Build history of the part. All positions in model axes, mm. Face numbers are marked on the shaded views. A direction names the side the tool comes from. Round coordinates to 2 decimals unless told otherwise and drop trailing zeros. Order: outer loops, then holes, each group sorted by start corner. A loop starts at its lowest first (then second) coordinate and runs counter-clockwise, first axis right, second up. Notation, with made-up numbers: M 87,-13.75 L 116,-13.75 A28 cw 116,23.25 Z; hole C 43.5,74 d6. An arc over 180 degrees is marked long. Use CSV: the item, a comma, the result in double quotes.
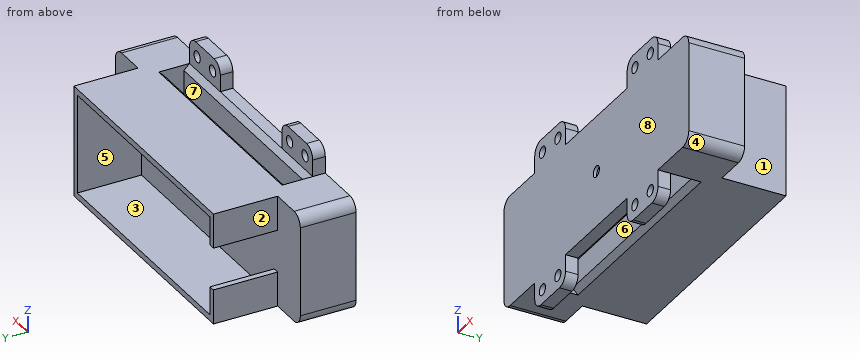
from build123d import *

# Parameters (mm, degrees)
SKETCH1_W            = 60
SKETCH1_H            = 20
BASE_DEPTH           = 10
SKETCH5_W            = 40
SKETCH5_H            = 3.5
CUT_EXTRUDE3_DEPTH   = 20
SKETCH6_W            = 40
SKETCH6_H            = 5
BOSS_EXTRUDE4_DEPTH  = 1
SKETCH8_W            = 40
SKETCH8_H            = 5
CUT_EXTRUDE6_DEPTH   = 1
CHAMFER2_SIZE        = 1
SKETCH13_W           = 45.3
SKETCH13_H           = 20
SKETCH13_W_2         = 43.1
SKETCH13_H_2         = 17.8
BOSS_EXTRUDE5_DEPTH  = 11.5
SKETCH14_W           = 3.171036328
SKETCH14_H           = 7.6
CUT_EXTRUDE11_DEPTH  = 11.5
FILLET2_R            = 2
SKETCH17_W           = 10
SKETCH17_H           = 2.25
BOSS_EXTRUDE7_DEPTH  = 5
SKETCH18_R           = 1
CUT_EXTRUDE12_DEPTH  = 2.25
FILLET3_R            = 2
FILLET3_OF_MIRROR6_R = 2
MIRROR7_OUTLINE_R    = 1
MIRROR7_DEPTH        = 2.25
SKETCH19_R           = 1
CUT_EXTRUDE13_DEPTH  = 0.6


# Read off the part's stored shape, not the designer's step: Mirror7
with BuildPart() as part:
    # Sketch1 → Base (new body)
    with BuildSketch(Plane(origin=(0, 0, 0), x_dir=(1, 0, 0), z_dir=(0, 1, 0))):
        Rectangle(SKETCH1_W, SKETCH1_H)
    extrude(amount=BASE_DEPTH)

    # Sketch5 → Cut-Extrude3 (cut)
    with BuildSketch(Plane(origin=(0, 0, -10), x_dir=(-1, 0, 0), z_dir=(0, 0, -1))):
        with Locations((0, 5)):
            Rectangle(SKETCH5_W, SKETCH5_H)
    extrude(amount=-CUT_EXTRUDE3_DEPTH, mode=Mode.SUBTRACT)

    # Sketch6 → Boss-Extrude4 (add)
    with BuildSketch(Plane(origin=(0, 3.25, 0), x_dir=(1, 0, 0), z_dir=(0, 1, 0))):
        Rectangle(SKETCH6_W, SKETCH6_H)
    extrude(amount=BOSS_EXTRUDE4_DEPTH)

    # Sketch8 → Cut-Extrude6 (cut)
    with BuildSketch(Plane.XZ.offset(-6.75)):
        Rectangle(SKETCH8_W, SKETCH8_H)
    extrude(amount=-CUT_EXTRUDE6_DEPTH, mode=Mode.SUBTRACT)

    # Chamfer2
    chamfer2_edges = [part.edges().sort_by_distance(p)[0] for p in [
        (0, 6.75, -2.5),
        (0, 6.75, 10),
        (0, 3.25, -2.5),
        (0, 3.25, 2.5),
        (0, 3.25, -10),
        (0, 6.75, -10),
        (0, 3.25, 10),
        (0, 6.75, 2.5),
    ]]
    chamfer(chamfer2_edges, length=CHAMFER2_SIZE - 0.0001)  # a hair under: the kernel refuses the full size

    # Sketch13 → Boss-Extrude5 (add)
    with BuildSketch(Plane(origin=(0, 10, 0), x_dir=(1, 0, 0), z_dir=(0, 1, 0))):
        Rectangle(SKETCH13_W, SKETCH13_H)
        Rectangle(SKETCH13_W_2, SKETCH13_H_2, mode=Mode.SUBTRACT)
    extrude(amount=BOSS_EXTRUDE5_DEPTH)

    # Sketch14 → Cut-Extrude11 (cut)
    with BuildSketch(Plane(origin=(0, 21.5, 0), x_dir=(1, 0, 0), z_dir=(0, 1, 0))):
        with Locations((-21.55, 0)):
            Rectangle(SKETCH14_W, SKETCH14_H)
    extrude(amount=-CUT_EXTRUDE11_DEPTH, mode=Mode.SUBTRACT)

    # Fillet2
    fillet2_edges = [part.edges().sort_by_distance(p)[0] for p in [
        (30, 5, 10),
        (-30, 5, 10),
        (-30, 5, -10),
        (30, 5, -10),
    ]]
    fillet(fillet2_edges, radius=FILLET2_R)

    # Sketch17 → Boss-Extrude7 (add)
    with BuildSketch(Plane.XY.offset(10)):
        with Locations((-15, 1.125)):
            Rectangle(SKETCH17_W, SKETCH17_H)
    boss_extrude7 = extrude(amount=BOSS_EXTRUDE7_DEPTH)

    # Sketch18 → Cut-Extrude12 (cut)
    with BuildSketch(Plane(origin=(0, 2.25, 0), x_dir=(1, 0, 0), z_dir=(0, 1, 0))):
        with Locations(Location((-17.5, -12.5, 0), (0, 0, 270))):
            Circle(SKETCH18_R)
        with Locations(Location((-12.5, -12.5, 0), (0, 0, 270))):
            Circle(SKETCH18_R)
    cut_extrude12 = extrude(amount=-CUT_EXTRUDE12_DEPTH, mode=Mode.SUBTRACT)

    # Fillet3
    fillet3_edges = [part.edges().sort_by_distance(p)[0] for p in [
        (-20, 1.125, 15),
        (-10, 1.125, 15),
    ]]
    fillet(fillet3_edges, radius=FILLET3_R)

    # Mirror6: Boss-Extrude7, Cut-Extrude12 across plane
    add(boss_extrude7.mirror(Plane(origin=(0, 0, 0), x_dir=(0, 0, 1), z_dir=(1, 0, 0))))
    add(cut_extrude12.mirror(Plane(origin=(0, 0, 0), x_dir=(0, 0, 1), z_dir=(1, 0, 0))), mode=Mode.SUBTRACT)

    # Fillet3 of Mirror6
    fillet3_of_mirror6_edges = [part.edges().sort_by_distance(p)[0] for p in [
        (20, 1.125, 15),
        (10, 1.125, 15),
    ]]
    fillet(fillet3_of_mirror6_edges, radius=FILLET3_OF_MIRROR6_R)

    # Mirror7 outline → Mirror7 (add)
    # profile 1 of 2: a face of its own
    with BuildSketch(Plane(origin=(0, 0, 0), x_dir=(1, 0, 0), z_dir=(0, 1, 0))):
        with BuildLine():
            ThreePointArc((-18, 15), (-19.414213562, 14.414213562), (-20, 13))
            Line((-20, 13), (-20, 10))
            Line((-20, 10), (-10, 10))
            Line((-10, 10), (-10, 13))
            ThreePointArc((-10, 13), (-10.585786438, 14.414213562), (-12, 15))
            Line((-12, 15), (-18, 15))
        make_face()
        with Locations((-17.5, 12.5)):
            Circle(MIRROR7_OUTLINE_R, mode=Mode.SUBTRACT)
        with Locations((-12.5, 12.5)):
            Circle(MIRROR7_OUTLINE_R, mode=Mode.SUBTRACT)
    # profile 2 of 2: a face of its own
    with BuildSketch(Plane(origin=(0, 0, 0), x_dir=(1, 0, 0), z_dir=(0, 1, 0))):
        with BuildLine():
            Line((10, 13), (10, 10))
            Line((10, 10), (20, 10))
            Line((20, 10), (20, 13))
            ThreePointArc((20, 13), (19.414213562, 14.414213562), (18, 15))
            Line((18, 15), (12, 15))
            ThreePointArc((12, 15), (10.585786438, 14.414213562), (10, 13))
        make_face()
        with Locations((12.5, 12.5)):
            Circle(MIRROR7_OUTLINE_R, mode=Mode.SUBTRACT)
        with Locations((17.5, 12.5)):
            Circle(MIRROR7_OUTLINE_R, mode=Mode.SUBTRACT)
    extrude(amount=MIRROR7_DEPTH)

    # Sketch19 → Cut-Extrude13 (cut)
    with BuildSketch(Plane.XZ):
        with Locations(Location((0, 0, 0), (0, 0, 270))):
            Circle(SKETCH19_R)
    extrude(amount=-CUT_EXTRUDE13_DEPTH, mode=Mode.SUBTRACT)


solid = part.part
(1) Cut at B-B, the plane z = 0. Give the cut face in (x, y), and give its area (3 significant figures).
Answer block:
outline,"M -30,0 L -1,0 L -1,0.6 L 1,0.6 L 1,0 L 30,0 L 30,10 L 22.65,10 L 22.65,21.5 L 21.55,21.5 L 21.55,10 L -30,10 Z; hole M -20,4.25 L 20,4.25 L 20,7.75 L -20,7.75 Z"
area,"471 mm²"
(2) Drop flat-ended pins along their axis: pin 1 (12 mm diameter, centred on x = -4, y = 8.5, fed in from +Z); pin 2 (2.5 mm diameter, centred on x = -12.5, z = 12.5, fed in from +Y); pin 3 (2.5 mm diameter, centred on y = 18, z = -7, fed in from +X). Give the stop position or say it passes through.
Answer block:
pin 1,"stops at z = 10"
pin 2,"stops at y = 2.25"
pin 3,"stops at x = 22.65"
(3) Tool access for the marked faces 1, 2, 3 and 4: list every direction of +Z, -Z, +X, -X, +Y, -Y with a clear straight run to the whole face (end or side of a thin tool).
Answer block:
face 1,"+Z, -Z, +X, +Y"
face 2,"+Z, -Z, -X, +Y"
face 3,"+Y"
face 4,"-Z, +X, +Y, -Y"
(4) Two-plate mould, pull along Y, no slides. Class the marked faces 5, 6, 7 and 8: released by +Y, released by -Y, zero draft, split by the parting line, or undercut.
Answer block:
face 5,"zero draft"
face 6,"undercut"
face 7,"undercut"
face 8,"released by -Y"
(5) Wall check: line 1 (Z direction, x = 12.5, y = 1.35); line 2 (X direction, y = 1.75, z = -12.5); line 3 (Z direction, x = -2, y = 16.75). Give the ranges that are in metal, low to high. Write a range as from..to.
Answer block:
line 1,"z = -15..-13.5, -11.5..11.5, 13.5..15"
line 2,"x = -20..-18.5, -16.5..-13.5, -11.5..-10, 10..11.5, 13.5..16.5, 18.5..20"
line 3,"z = -10..-8.9, 8.9..10"
(6) Cut at C-C, the plane y = 15.75. Give the cut face in (x, z), and give its area (3 significant figures).
Answer block:
outline,"M -22.65,-10 L 22.65,-10 L 22.65,10 L -22.65,10 L -22.65,3.8 L -21.55,3.8 L -21.55,8.9 L 21.55,8.9 L 21.55,-8.9 L -21.55,-8.9 L -21.55,-3.8 L -22.65,-3.8 Z"
area,"130 mm²"
